Model file for the job. Use its own axes, mm. Face numbers are marked on the shaded views. A direction names the side the tool comes from. Give positions to 0.01 mm unless a question says otherwise; leave off trailing zeros. Loops run counter-clockwise (first coordinate to the right, second up) from the corner with the lowest first, then second, coordinate; pieces in that order, holes last. Notation, with made-up numbers: (60, -22) - (76, -22) arc R20 cw to (76, -14) - close; hole circle Ø1 at (68, 29). An arc over 180 degrees is marked (long way). Use a Markdown table: item, result.
from build123d import *

# Parameters (mm, degrees)
F1_DEPTH = 35.56
F3_DEPTH = 5.08


with BuildPart() as f1:
    # F0 (on Top) → F1 (new body)
    with BuildSketch(Plane.XY):
        with BuildLine():
            ThreePointArc((10.998523, 6.35), (0, -12.7), (-10.998523, 6.35))
            Line((-10.998523, 6.35), (-13.198227, 7.62))
            ThreePointArc((-13.198227, 7.62), (0, -15.24), (13.198227, 7.62))
            Line((13.198227, 7.62), (10.998523, 6.35))
        make_face()
    extrude(amount=F1_DEPTH)

    # F2 (on Top) → F3 (join)
    with BuildSketch(Plane.XY):
        with BuildLine():
            Line((22.86, 0), (15.24, 0))
            ThreePointArc((15.24, 0), (0, -15.24), (-15.24, 0))
            Line((-15.24, 0), (-22.86, 0))
            Line((-22.86, 0), (-22.86, -17.78))
            Line((-22.86, -17.78), (0, -17.78))
            Line((0, -17.78), (22.86, -17.78))
            Line((22.86, -17.78), (22.86, 0))
        make_face()
    extrude(amount=F3_DEPTH)


solid = f1.part
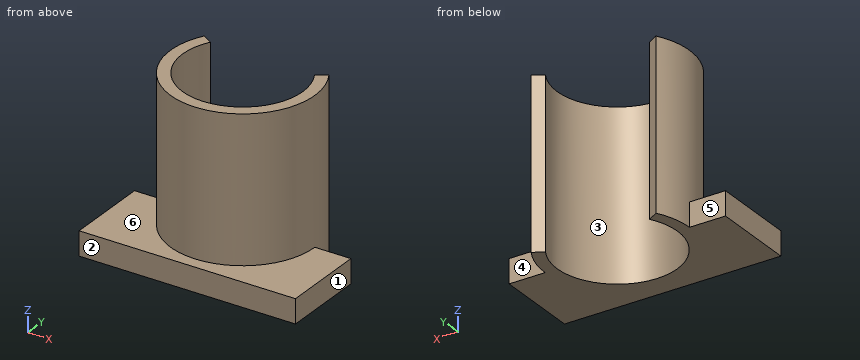
(1) 3-axis set-ups, long thin cutter, end or side, ignore diameter. For the marked faces 4, 5 and 6: which of +Z, -Z, +X, -X, +Y, -Y reach the whole face in a straight line?
Computed:
| item | result |
|---|---|
| face 4 | +Z, -Z, +X, +Y |
| face 5 | +Z, -Z, -X, +Y |
| face 6 | +Z, -Y |
(2) Slice it at D-D, the plane y = 2.5. Write the cut outline in (x, z).
Computed:
| item | result |
|---|---|
| outline | (-15.03, 0) - (-12.45, 0) - (-12.45, 35.56) - (-15.03, 35.56) - close; (12.45, 0) - (15.03, 0) - (15.03, 35.56) - (12.45, 35.56) - close |
(3) Mould opens along Y. For the marked faces 1, 2 and 3 say: pulls with the +Y half, pulls with the -Y half, needs draft (parallel to the pull), parting line crosses it, or undercut.
Computed:
| item | result |
|---|---|
| face 1 | needs draft |
| face 2 | pulls with the -Y half |
| face 3 | undercut |
(4) Slice it at C-C, the plane x = 0. Write the cut outline in (y, z), plus the area to 3 significant figures.
Computed:
| item | result |
|---|---|
| outline | (-17.78, 0) - (-12.7, 0) - (-12.7, 35.56) - (-15.24, 35.56) - (-15.24, 5.08) - (-17.78, 5.08) - close |
| area | 103 mm² |
(5) Drill centre lines: probe 1 along X at (y, z) = (0, 9.5); probe 2 along Z at (x, y) = (-5.5, -16.25); probe 3 along Y at (x, z) = (0, 16.5). Where is each one in solid material? Low to high. Write a range as [from, to].
Computed:
| item | result |
|---|---|
| probe 1 | [-15.24, -12.7], [12.7, 15.24] |
| probe 2 | [0, 5.08] |
| probe 3 | [-15.24, -12.7] |
(6) Slice it at A-A, the plane y = -8. Write the cut outline in (x, z), plus the area to 3 significant figures.
Computed:
| item | result |
|---|---|
| outline | (-22.86, 0) - (-9.86, 0) - (-9.86, 35.56) - (-12.97, 35.56) - (-12.97, 5.08) - (-22.86, 5.08) - close; (9.86, 0) - (22.86, 0) - (22.86, 5.08) - (12.97, 5.08) - (12.97, 35.56) - (9.86, 35.56) - close |
| area | 321 mm² |
(7) Slice it at B-B, the plane z = 2.5. Write the cut outline in (x, y).
Computed:
| item | result |
|---|---|
| outline | (-22.86, -17.78) - (22.86, -17.78) - (22.86, 0) - (15.24, 0) arc R15.24 ccw to (13.2, 7.62) - (11, 6.35) arc R12.7 cw (long way) to (-11, 6.35) - (-13.2, 7.62) arc R15.24 ccw to (-15.24, 0) - (-22.86, 0) - close |
(8) Pin check, flat tips, straight feed: P1, Ø2.5, axis at x = -18.5, z = 2.5, coming from the +Y side; P2, Ø6, axis at y = -12.5, z = 11, coming from the +X side; P3, Ø4, axis at y = -15, z = 22, coming from the +X side; P4, Ø4, axis at x = -5.5, y = -15, coming from the +Z side. Stop position of each tip, or through.
Computed:
| item | result |
|---|---|
| P1 | y = 0 |
| P2 | x = 11.92 |
| P3 | x = 7.95 |
| P4 | z = 35.56 |
